For this review, take the finished solid that the model builds, in its own axes (mm). Give positions to 0.01 mm unless a question says otherwise; leave off trailing zeros. Loops run counter-clockwise (first coordinate to the right, second up) from the corner with the lowest first, then second, coordinate; pieces in that order, holes last.
Autodesk Inventor part; units mm, degrees
ref_plane "Work Plane1" through (29, 0, 0) normal (0, -1, 0) x (1, 0, 0)
ref_plane "YZ Plane" through (0, 0, 0) normal (1, 0, 0) x (0, 1, 0)
ref_plane "XZ Plane" through (0, 0, 0) normal (0, 1, 0) x (-1, 0, 0)
sketch "Sketch1" plane through (0, 0, 0) normal (0, 0, 1) x (1, 0, 0)
  line L0 (0.1439, 0) -> (6.35, 0)
  line L1 (6.35, 0) -> (6.35, 0.9271)
  line L2 (6.35, 0.9271) -> (0.7927, 0.9271)
  line L3 (0.7927, 0.9271) -> (0.0001, 0.9271)
  line L4 (0.0001, 0.9271) -> (0, 0.9271)
  line L5 (0, 0.9271) -> (0, 1.7653)
  line L6 (0, 1.7653) -> (-0.9906, 1.7653)
  line L7 (-0.9906, 1.7653) -> (-0.9906, 0.7332)
  line L8 (-0.9906, 0.7332) -> (-0.2794, 0.7332)
  line L9 (-0.2794, 0.7332) -> (0.1439, 0)
  line L10 (-2.4587, 0) -> (7.8181, 0)
  line L11 (0, -0.3531) -> (0, 2.1184)
  line L12 (0.7927, 0.9271) -> (0, 0.9271) construction
  dimension "d1" = 5.5573
  dimension "d2" = 0.7926
  dimension "d3" = 0.9906
  dimension "d4" = 0.7112
  dimension "d5" = 60
  dimension "d6" = 1.8542
  dimension "d7" = 1.8542
  dimension "d8" = 1.4665
  dimension "d9" = 3.5306
  dimension "d26" = 6.35
revolve "Body" add sketch "Sketch1" angle 360 about axis through (0.1439, 0, 0) along (1, 0, 0) contours L9 L11 L3 L2 L1 L0 | L9 L8 L7 L6 L5 L11
sketch "Sketch2" plane through (-0.9906, 0, 0) normal (-1, 0, 0) x (0, 0, 1)
  circle A0 centre (0, 0) radius 0.7332
  line L0 (0, -2.4714) -> (0, 2.4714)
  line L1 (-2.4714, 0) -> (2.4714, 0)
  line L2 (0.7332, 0) -> (0.3666, -0.635)
  line L3 (0.3666, -0.635) -> (-0.3666, -0.635)
  line L4 (-0.3666, -0.635) -> (-0.7332, 0)
  line L5 (-0.7332, 0) -> (-0.3666, 0.635)
  line L6 (-0.3666, 0.635) -> (0.3666, 0.635)
  line L7 (0.3666, 0.635) -> (0.7332, 0)
  point P0 (0, 0)
extrude "Slot" add sketch "Sketch2" against normal up to next contours L7 A0 | A0 L2 | L6 L0 A0 | A0 L0 L3 | L0 L6 A0 | A0 L3 L0 | L4 A0 | A0 L5
fillet "Fillet1" radius 0.9905 1 edges at (-0.9906, -1.7653, 0)
thread "Thread"
chamfer "Chamfer1" distance 0.2435 distance2 0.2433 1 edges at (6.35, -0.9271, 0) measured on face at (6.35, -0.6833, -0.2193)
ref_plane "Work Plane1" through (29, 0, 0) normal (0, -1, 0) x (1, 0, 0)
fillet "Fillet2" radius 0.1 1 edges at (0.0001, -0.9271, 0)
equation "\"d1\" = GEL"
equation "\"d3\" = KOH"
equation "\"d4\" = INTI"
equation "\"d6\" = GD"
equation "\"d7\" = BDM"
equation "\"d8\" = 1.1547 * SW"
equation "\"d9\" = KOD"
equation "\"d26\" = NLG"
equation "\"d30\" = R"
equation "\"d17\" = RR"
equation "\"d13\" = GEL"
equation "\"d15\" = -0.5 * SPD + 0.5 * GD"
equation "\"d16\" = GUL"
equation "\"GD\" = NND"
equation "\"NLG\" = 6.35"
equation "\"GEL\" = 5.55732"
equation "\"KOD\" = 3.5306"
equation "\"KOH\" = 0.9906"
equation "\"INTI\" = 0.7112"
equation "\"GAL\" = 0.79248"
equation "\"GUL\" = 0.24333"
equation "\"BDM\" = NND"
equation "\"SW\" = 1.27"
equation "\"RR\" = 0.9905"
equation "\"SPD\" = 1.36728"
equation "\"R\" = 0.1"
equation "\"TOA\" = 30deg"
equation "\"GD1\" = SPD"
equation "\"THREADDIA\" = 1.8542"
equation "\"KOH1\" = 0.254"
equation "\"NND\" = 1.8542"
equation "\"E0\" = 1.46685"
properties part number "ANSI B18.3 - 1 - 64 x 1/4"
Q1. For probe 1 along X at (y, z) = (-0.8, 0.4); probe 2 along Y at (x, z) = (2, -0.75) (3 decimals); probe 3 along Z at (x, y) = (6, -0.65), list the stretches that pass through material, from the lowest coordinate up.
Answers:
probe 1: x = -0.98 to 6.14
probe 2: y = -0.545 to 0.545
probe 3: z = -0.66 to 0.66
Q2. Mouldability with a two-part tool opening along Z and no side actions: class faces 1 (the cylindrical face through (3.06, 0.43, 0.82)), 2 (the flat face through (6.35, 0, 0)), 3 (the conical face through (0.12, -0.01, 0.04)) as +Z half, -Z half, draft (parallel to the pull), parting line (faces both ways), or undercut.
Answers:
face 1: parting line
face 2: draft
face 3: undercut
Q3. Consider section A-A on x = 5.75. Give the boundary of the cut face in (y, z).
Answers:
outline: circle Ø1.85 at (0, 0)
Q4. For pin 1 Ø1 at (x, z) = (4.5, 1) entering from -Y, flat-tipped, find the tip position at first contact; note if it passes through.
Answers:
pin 1: stops at y = -0.78
